```python
from build123d import *

# Parameters (mm, degrees)
F0_W     = 107.602417469
F0_H     = 87.8107035317
F1_DEPTH = 81


# Not quite as in the source:
# - ends of sketch curves that miss each other by under 0.0002 mm in the source are joined


with BuildPart() as f1:
    # F0 (on Top) → F1 (new body)
    with BuildSketch(Plane.XY):
        Rectangle(F0_W, F0_H)
        with BuildLine():
            Line((-43.4592129171, -38.9053517658), (-48.8012087345, -38.9053517658))
            Line((-48.8012087345, -38.9053517658), (-48.8012087345, -18.2926106175))
            ThreePointArc((-48.8012087345, -18.2926106175), (-45.2040241526, -22.3437425741), (-43.9055000032, -27.6035184325))
            ThreePointArc((-43.9055000032, -27.6035184325), (-42.8947395838, -33.2544350992), (-39.987798415, -38.2046056862))
            ThreePointArc((-39.987798415, -38.2046056862), (-39.6614460497, -38.566308994), (-39.3116101623, -38.9053517658))
            Line((-39.3116101623, -38.9053517658), (-43.4592129171, -38.9053517658))
        make_face(mode=Mode.SUBTRACT)
        with BuildLine():
            ThreePointArc((-38.9055000032, -27.6035184325), (-40.0867237079, -21.511151528), (-43.4592129171, -16.3016850991))
            Line((-43.4592129171, -16.3016850991), (-11.748120417, -16.3016850991))
            ThreePointArc((-11.748120417, -16.3016850991), (-15.120609628, -21.5111515275), (-16.3018333334, -27.6035184325))
            ThreePointArc((-16.3018333334, -27.6035184325), (-27.6036666683, -38.9053517674), (-38.9055000032, -27.6035184325))
        make_face(mode=Mode.SUBTRACT)
        with BuildLine():
            Line((-43.4586830682, -11.3016850991), (-48.8012087345, -11.3016850991))
            Line((-48.8012087345, -11.3016850991), (-48.8012087345, 9.3111358172))
            ThreePointArc((-48.8012087345, 9.3111358172), (-45.2037061615, 5.2599802444), (-43.9050552974, 0))
            ThreePointArc((-43.9050552974, 0), (-42.7238541219, -6.0922822479), (-39.3514275267, -11.3016850991))
            Line((-39.3514275267, -11.3016850991), (-43.4586830682, -11.3016850991))
        make_face(mode=Mode.SUBTRACT)
        with BuildLine():
            ThreePointArc((-11.3018333334, -27.6035184325), (0, -16.3016850991), (11.3018333333, -27.6035184325))
            ThreePointArc((11.3018333334, -27.6035184325), (12.4830570387, -33.6958853375), (15.8555462497, -38.9053517658))
            Line((15.8555462497, -38.9053517658), (-15.8555462474, -38.9053517658))
            ThreePointArc((-15.8555462474, -38.9053517658), (-12.4830570378, -33.6958853372), (-11.3018333334, -27.6035184325))
        make_face(mode=Mode.SUBTRACT)
        with BuildLine():
            ThreePointArc((38.9055, -27.6035184325), (27.6036666667, -38.9053517658), (16.3018333334, -27.6035184325))
            ThreePointArc((16.3018333334, -27.6035184325), (15.120609628, -21.5111515275), (11.748120417, -16.3016850991))
            Line((11.748120417, -16.3016850991), (43.4592129164, -16.3016850991))
            ThreePointArc((43.4592129164, -16.3016850991), (40.0867237054, -21.5111515275), (38.9055, -27.6035184325))
        make_face(mode=Mode.SUBTRACT)
        with BuildLine():
            ThreePointArc((43.9055, -27.6035184325), (45.2040241503, -22.3437425739), (48.8012087345, -18.2926106186))
            Line((48.8012087345, -18.2926106186), (48.8012087345, -38.9053517658))
            Line((48.8012087345, -38.9053517658), (43.4592129164, -38.9053517658))
            Line((43.4592129164, -38.9053517658), (39.3517870837, -38.9053517658))
            ThreePointArc((39.3517870837, -38.9053517658), (42.7242762947, -33.6958853375), (43.9055, -27.6035184325))
        make_face(mode=Mode.SUBTRACT)
        with BuildLine():
            Line((15.855319758, 11.3016850991), (43.4586830625, 11.3016850991))
            ThreePointArc((43.4586830625, 11.3016850991), (40.0862564691, 6.0922822475), (38.9050552942, 0))
            ThreePointArc((38.9050553006, 0), (27.6033701999, -11.3016851007), (16.3016850991, 0))
            ThreePointArc((16.3016850991, 0), (15.1204839236, 6.0922822479), (11.7480573284, 11.3016850991))
            Line((11.7480573284, 11.3016850991), (15.855319758, 11.3016850991))
        make_face(mode=Mode.SUBTRACT)
        with BuildLine():
            ThreePointArc((43.9050552942, 0), (45.2037061591, 5.2599802476), (48.8012087345, 9.3111358227))
            Line((48.8012087345, 9.3111358227), (48.8012087345, -11.3016850991))
            Line((48.8012087345, -11.3016850991), (43.4586830625, -11.3016850991))
            Line((43.4586830625, -11.3016850991), (39.3514275289, -11.3016850991))
            ThreePointArc((39.3514275289, -11.3016850991), (42.7238548196, -6.0922824277), (43.9050552942, 0))
        make_face(mode=Mode.SUBTRACT)
        with BuildLine():
            ThreePointArc((-16.3016850991, 0), (-27.6033701983, -11.3016850991), (-38.9050552974, 0))
            ThreePointArc((-38.9050552974, 0), (-40.086256473, 6.0922822479), (-43.4586830682, 11.3016850991))
            Line((-43.4586830682, 11.3016850991), (-15.8553128699, 11.3016850991))
            Line((-15.8553128699, 11.3016850991), (-11.7480573284, 11.3016850991))
            ThreePointArc((-11.7480573284, 11.3016850991), (-15.1204839236, 6.0922822479), (-16.3016850991, 0))
        make_face(mode=Mode.SUBTRACT)
        with BuildLine():
            Line((-48.8012087345, 16.3016850991), (-48.8012087345, 36.9144262464))
            ThreePointArc((-48.8012087345, 36.9144262464), (-45.2040241503, 32.8632942911), (-43.9055, 27.6035184325))
            ThreePointArc((-43.9055, 27.6035184325), (-42.7242762947, 21.5111515275), (-39.3517870837, 16.3016850991))
            Line((-39.3517870837, 16.3016850991), (-43.4592129164, 16.3016850991))
            Line((-43.4592129164, 16.3016850991), (-48.8012087345, 16.3016850991))
        make_face(mode=Mode.SUBTRACT)
        with BuildLine():
            ThreePointArc((-38.9055, 27.6035184325), (-40.0867237054, 33.6958853375), (-43.4592129164, 38.9053517658))
            Line((-43.4592129164, 38.9053517658), (-15.8555462497, 38.9053517658))
            Line((-15.8555462497, 38.9053517658), (-11.748120417, 38.9053517658))
            ThreePointArc((-11.748120417, 38.9053517658), (-15.120609628, 33.6958853375), (-16.3018333334, 27.6035184325))
            ThreePointArc((-16.3018333334, 27.6035184325), (-27.6036666667, 16.3016850991), (-38.9055, 27.6035184325))
        make_face(mode=Mode.SUBTRACT)
        with BuildLine():
            ThreePointArc((-11.3016850991, 0), (0, 11.3016850991), (11.3016850991, 0))
            ThreePointArc((11.3016850991, 0), (12.4805105623, -6.0863826289), (15.8464978932, -11.2925148079))
            ThreePointArc((15.8464978932, -11.2925148079), (15.8510483075, -11.2971849132), (15.8557668328, -11.3016850991))
            Line((15.8557668328, -11.3016850991), (-15.8553128699, -11.3016850991))
            ThreePointArc((-15.8553128699, -11.3016850991), (-12.4828862747, -6.0922822479), (-11.3016850991, 0))
        make_face(mode=Mode.SUBTRACT)
        with BuildLine():
            ThreePointArc((-11.3018333334, 27.6035184325), (0, 38.9053517658), (11.3018333334, 27.6035184325))
            ThreePointArc((11.3018333334, 27.6035184325), (12.4806822619, 21.5170487891), (15.8467347518, 16.310851698))
            ThreePointArc((15.8467347518, 16.310851698), (15.8512041563, 16.3060464442), (15.8561076969, 16.3016850991))
            Line((15.8561076969, 16.3016850991), (-15.8555462497, 16.3016850991))
            ThreePointArc((-15.8555462497, 16.3016850991), (-12.4830570387, 21.5111515275), (-11.3018333334, 27.6035184325))
        make_face(mode=Mode.SUBTRACT)
        with BuildLine():
            ThreePointArc((38.9055, 27.6035184325), (27.6036666667, 16.3016850991), (16.3018333334, 27.6035184325))
            ThreePointArc((16.3018333334, 27.6035184325), (15.120609628, 33.6958853375), (11.748120417, 38.9053517658))
            Line((11.748120417, 38.9053517658), (15.8555462497, 38.9053517658))
            Line((15.8555462497, 38.9053517658), (43.4592129164, 38.9053517658))
            ThreePointArc((43.4592129164, 38.9053517658), (40.0867237054, 33.6958853375), (38.9055, 27.6035184325))
        make_face(mode=Mode.SUBTRACT)
        with BuildLine():
            ThreePointArc((43.9055, 27.6035184325), (45.2040241503, 32.8632942911), (48.8012087345, 36.9144262464))
            Line((48.8012087345, 36.9144262464), (48.8012087345, 27.6035184325))
            Line((48.8012087345, 27.6035184325), (48.8012087345, 16.3016850991))
            Line((48.8012087345, 16.3016850991), (43.4592129164, 16.3016850991))
            Line((43.4592129164, 16.3016850991), (39.3517870837, 16.3016850991))
            ThreePointArc((39.3517870837, 16.3016850991), (42.7242762947, 21.5111515275), (43.9055, 27.6035184325))
        make_face(mode=Mode.SUBTRACT)
    extrude(amount=F1_DEPTH)


solid = f1.part
```
Input: part model. Units: mm. Frame: model coordinates. A direction names the side the tool comes from. Give positions to 0.01 mm unless a question says otherwise; leave off trailing zeros. Order: outer loops, then holes, each group sorted by start corner. A loop starts at its lowest first (then second) coordinate and runs counter-clockwise, first axis right, second up. Notation, with made-up numbers: (28, 46) -> (51, 46) arc R10 ccw to (51, 63) -> close; hole circle Ø10 at (-13.5, -39.75). An arc over 180 degrees is marked (long way). Write each question's results on one line, items separated by ' | '. Start each with the question number.
Item 1: Cut plane C-C on z = 10. Give the number of separate pieces and of enclosed holes in the cut face, then the cut area to 3 significant figures.
Item 2: Cut plane D-D on x = -19. Return the cut outline in (y, z), then the cut area to 3 significant figures.
Item 3: Line query: line 1 (X direction, y = -34, z = 40); line 2 (Y direction, x = 26.5, z = 33.5); line 3 (X direction, y = -7.5, z = 33). Output: solid intervals per line, ascending.
Item 4: Cut plane A-A on x = 0. Return the cut outline in (y, z), then the cut area to 3 significant figures.
Item 5: Cut plane B-B on y = -34. Return the cut outline in (x, z), then the cut area to 3 significant figures.
Item 6: Set-up query: faces 3 (the flat face through (12, 3, 0)), 4 (the flat face through (-48.801, -1, 40)). Return all of +Z, -Z, +X, -X, +Y, -Y with unobstructed straight access to the full face (end or side cutting, diameter ignored); none if empty.
Item 7: Mould query, pull axis X, two halves, no side actions, for faces 1 (the flat face through (12, 3, 81)), 2 (the flat face through (44, -38.905, 40)). Classes: pulls with the +X half, pulls with the -X half, needs draft (parallel to the pull), parting line crosses it, or undercut.
Established:
1) separate pieces: 1 | enclosed holes: 15 | area: 4,430 mm^2
2) outline: (-43.91, 0) -> (-34.93, 0) -> (-34.93, 81) -> (-43.91, 81) -> close; (-16.3, 0) -> (-7.33, 0) -> (-7.33, 81) -> (-16.3, 81) -> close; (11.3, 0) -> (20.27, 0) -> (20.27, 81) -> (11.3, 81) -> close; (38.91, 0) -> (43.91, 0) -> (43.91, 81) -> (38.91, 81) -> close | area: 2,590 mm^2
3) line 1: -53.8 to -48.8, -42.6 to -36.92, -18.29 to -12.61, 12.61 to 18.29, 36.92 to 42.6, 48.8 to 53.8 | line 2: -43.91 to -38.85, -16.3 to -11.25, 11.3 to 16.36, 38.91 to 43.91 | line 3: -53.8 to -48.8, -42.08 to -36.06, -19.15 to -13.13, 13.13 to 19.15, 36.06 to 42.08, 48.8 to 53.8
4) outline: (-43.91, 0) -> (-38.91, 0) -> (-38.91, 81) -> (-43.91, 81) -> close; (-16.3, 0) -> (-11.3, 0) -> (-11.3, 81) -> (-16.3, 81) -> close; (11.3, 0) -> (16.3, 0) -> (16.3, 81) -> (11.3, 81) -> close; (38.91, 0) -> (43.91, 0) -> (43.91, 81) -> (38.91, 81) -> close | area: 1,620 mm^2
5) outline: (-53.8, 0) -> (-48.8, 0) -> (-48.8, 81) -> (-53.8, 81) -> close; (-42.6, 0) -> (-36.92, 0) -> (-36.92, 81) -> (-42.6, 81) -> close; (-18.29, 0) -> (-12.61, 0) -> (-12.61, 81) -> (-18.29, 81) -> close; (12.61, 0) -> (18.29, 0) -> (18.29, 81) -> (12.61, 81) -> close; (36.92, 0) -> (42.6, 0) -> (42.6, 81) -> (36.92, 81) -> close; (48.8, 0) -> (53.8, 0) -> (53.8, 81) -> (48.8, 81) -> close | area: 2,650 mm^2
6) face 3: -Z, +X, -X, +Y, -Y | face 4: +Z, -Z
7) face 1: needs draft | face 2: undercut
